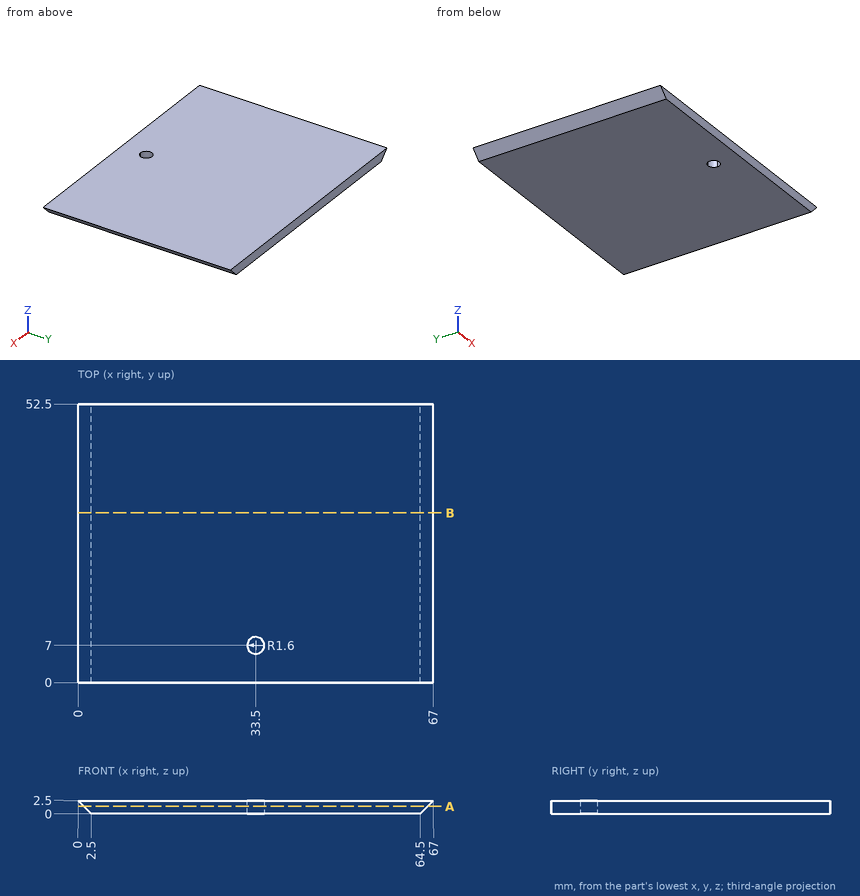
Source: three-view drawing plus pictorial views. Frame: mm from the lowest corner of the part. Coordinates: 2 decimals unless noted, no trailing zeros. Loops run counter-clockwise (first coordinate to the right, second up) from the corner with the lowest first, then second, coordinate; pieces in that order, holes last. Notation, with made-up numbers: (20, 57) -> (29, 57) arc R34 cw to (29, 89) -> close; hole circle Ø5 at (-12.5, -15). An arc over 180 degrees is marked (long way). Write each question's results on one line, items separated by ' | '. Start each with the question number.
Q1. Section B-B, the plane y = 32. Return the cut outline in (x, z), plus the area to 3 significant figures.
Q2. Section A-A, the plane z = 1.4. Return the cut outline in (x, y).
Q3. Ray query, line 1 (Y direction, x = 34.5, z = 0.85); line 2 (X direction, y = 7.5, z = 1.7); line 3 (X direction, y = 21, z = 0.7). Return the intervals inside material, ascending. Write a range as from..to.
Found:
1) outline: (0, 2.5) -> (2.5, 0) -> (64.5, 0) -> (67, 2.5) -> close | area: 161 mm2
2) outline: (1.1, 0) -> (65.9, 0) -> (65.9, 52.5) -> (1.1, 52.5) -> close; hole circle Ø3.2 at (33.5, 7)
3) line 1: 0..5.75, 8.25..52.5 | line 2: 0.8..31.98, 35.02..66.2 | line 3: 1.8..65.2
